Can you work these out from the model? Positions are in its coordinate system, mm. A direction names the side the tool comes from. Give positions to 0.01 mm unless a question says otherwise; leave off trailing zeros. Order: outer loops, then holes, each group sorted by start corner. A loop starts at its lowest first (then second) coordinate and runs counter-clockwise, first axis right, second up.
```python
from build123d import *

# Parameters (mm, degrees)
SKETCH1_R           = 2.5
SKETCH1_R_2         = 1.75
BOSS_EXTRUDE1_DEPTH = 4
SKETCH3_R           = 4.75
SKETCH3_R_2         = 1.75
BOSS_EXTRUDE2_DEPTH = 2.5
FILLET1_R           = 3
FILLET2_R           = 15
SKETCH4_R           = 1.75
CUT_EXTRUDE1_DEPTH  = 2.75


with BuildPart() as part:
    # Sketch1 → Boss-Extrude1 (new body)
    with BuildSketch(Plane(origin=(0, 0, 0), x_dir=(1, 0, 0), z_dir=(0, 1, 0))):
        with BuildLine():
            Line((-33.743770102, 11.787151842), (-29.558909379, 8.857749335))
            ThreePointArc((-29.558909379, 8.857749335), (-30.943257909, 1.876678146), (-29.553838003, -5.103385472))
            Line((-29.553838003, -5.103385472), (-33.733356926, -8.013259417))
            ThreePointArc((-33.733356926, -8.013259417), (-34.979887519, -14.973587102), (-28.019559835, -16.220117695))
            Line((-28.019559835, -16.220117695), (-11.208684115, -4.516012477))
            Line((-11.208684115, -4.516012477), (5.907787468, -4.516012477))
            ThreePointArc((5.907787468, -4.516012477), (10.657787468, 0.233987523), (5.907787468, 4.983987523))
            Line((5.907787468, 4.983987523), (-6.587027339, 4.983987523))
            Line((-6.587027339, 4.983987523), (-28.009146659, 19.979471047))
            ThreePointArc((-28.009146659, 19.979471047), (-34.972617983, 18.750623166), (-33.743770102, 11.787151842))
        make_face()
        with Locations((-30.87645838, 15.883311444)):
            Circle(SKETCH1_R, mode=Mode.SUBTRACT)
        with Locations((-30.87645838, -12.116688556)):
            Circle(SKETCH1_R, mode=Mode.SUBTRACT)
        with Locations((-26.092212532, 0.233987523)):
            Circle(SKETCH1_R_2, mode=Mode.SUBTRACT)
        with Locations((5.907787468, 0.233987523)):
            Circle(SKETCH1_R_2, mode=Mode.SUBTRACT)
    extrude(amount=BOSS_EXTRUDE1_DEPTH)

    # Sketch3 → Boss-Extrude2 (add)
    with BuildSketch(Plane(origin=(0, 4, 0), x_dir=(1, 0, 0), z_dir=(0, 1, 0))):
        with Locations((-26.092212532, 0.233987523)):
            Circle(SKETCH3_R)
        with Locations((-26.092212532, 0.233987523)):
            Circle(SKETCH3_R_2, mode=Mode.SUBTRACT)
        with Locations((5.907787468, 0.233987523)):
            Circle(SKETCH3_R)
        with Locations((5.907787468, 0.233987523)):
            Circle(SKETCH3_R_2, mode=Mode.SUBTRACT)
    extrude(amount=BOSS_EXTRUDE2_DEPTH)

    # Fillet1
    fillet1_edges = [part.edges().sort_by_distance(p)[0] for p in [
        (-29.553838003, 2, 5.103385472),
        (-29.558909379, 2, -8.857749335),
    ]]
    fillet(fillet1_edges, radius=FILLET1_R)

    # Fillet2
    fillet2_edges = [part.edges().sort_by_distance(p)[0] for p in [
        (-11.208684115, 2, 4.516012477),
        (-6.587027339, 2, -4.983987523),
    ]]
    fillet(fillet2_edges, radius=FILLET2_R)

    # Sketch4 → Cut-Extrude1 (cut)
    with BuildSketch(Plane.XZ):
        with BuildLine():
            ThreePointArc((-2.629044497, 2.616012477), (-3.092212532, -0.233987523), (-2.629044497, -3.083987523))
            Line((-2.629044497, -3.083987523), (9.707787468, -3.083987523))
            ThreePointArc((9.707787468, -3.083987523), (10.657787468, -0.233987523), (9.707787468, 2.616012477))
            Line((9.707787468, 2.616012477), (-2.629044497, 2.616012477))
        make_face()
        with Locations((5.907787468, -0.233987523)):
            Circle(SKETCH4_R, mode=Mode.SUBTRACT)
        with BuildLine():
            Line((-30.90374362, -3.083987523), (-17.555380567, -3.083987523))
            ThreePointArc((-17.555380567, -3.083987523), (-17.092212532, -0.233987523), (-17.555380567, 2.616012477))
            Line((-17.555380567, 2.616012477), (-30.380287253, 2.616012477))
            ThreePointArc((-30.380287253, 2.616012477), (-30.866740114, -0.213350056), (-30.90374362, -3.083987523))
        make_face()
        with Locations((-26.092212532, -0.233987523)):
            Circle(SKETCH4_R, mode=Mode.SUBTRACT)
    extrude(amount=-CUT_EXTRUDE1_DEPTH, mode=Mode.SUBTRACT)


solid = part.part
```
1) Which directions (+Z, -Z, +X, -X, +Y, -Y) give clear straight access to the entire face, cutting with the end or side of a thin tool? Please do faces 1 (the face through (-24, 2.75, 0)), 2 (the face through (-21.704, 5.232, 1.585)), 3 (the face through (-32.559, 1.972, 7.195)).
2) Suppose I cut it at C-C (y = 5.5). Please give me the cut outline in (x, z).
3) Suppose I cut it at D-D (y = 1.5). Please give me the cut outline in (x, z).
4) We'd pull the mould along X, two halves only. Please class faces 4 (the face through (-19.9, 0, -3.4)), 5 (the face through (10.1, 3.9, 2)), 6 (the face through (-35.042, 1.972, 14.883)): +X half, -X half, draft (parallel to the pull), parting line (faces both ways), or undercut.
5) Suppose I cut it at B-B (x = -26). Please give me the cut outline in (y, z).
6) If I drill on line 1 (X direction, y = 6, z = 1); line 2 (Y direction, x = -25, z = -14); line 3 (Z direction, x = 3, y = 3.75), over which ranges is the centre line in solid material (lowest first)?
7) Suppose I cut it at A-A (z = -17.5). Please give me the cut outline in (x, y), and give its area (3 significant figures).
8) I'm going to push flat-ended pins straight in: pin 1 Ø8 at (x, z) = (-30.88, 12.12) entering from +Y; pin 2 Ø3 at (x, y) = (-23.5, 1.5) entering from -Z; pin 3 Ø2 at (x, y) = (-16, 3) entering from +Z; pin 4 Ø3 at (x, z) = (-30.88, -15.88) entering from +Y. Where does each tip first touch, or does it pass through?
Results:
1. face 1: -X, -Y
1. face 2: +Y
1. face 3: -X, +Y, -Y
2. outline: circle Ø9.5 at (-26.09, -0.23); circle Ø9.5 at (5.91, -0.23); hole circle Ø3.5 at (-26.09, -0.23); hole circle Ø3.5 at (5.91, -0.23)
3. outline: (-33.74, -11.79) arc R5 ccw to (-28.01, -19.98) - (-10.46, -7.7) arc R15 cw to (-1.86, -4.98) - (5.91, -4.98) arc R4.75 ccw to (9.71, -3.08) - (-2.63, -3.08) arc R9 cw to (-2.63, 2.62) - (9.71, 2.62) arc R4.75 ccw to (5.91, 4.52) - (-6.5, 4.52) arc R15 cw to (-15.07, 7.21) - (-28.02, 16.22) arc R5 ccw to (-33.73, 8.01) - (-31.42, 6.4) arc R3 cw to (-30.25, 3.12) arc R18.26 ccw to (-30.38, 2.62) - (-17.56, 2.62) arc R9 cw to (-17.56, -3.08) - (-30.9, -3.08) arc R18.26 ccw to (-30.25, -6.88) arc R3 cw to (-31.41, -10.16) - close; hole circle Ø5 at (-30.88, -15.88); hole circle Ø5 at (-30.88, 12.12)
4. face 4: draft
4. face 5: undercut
4. face 6: parting line
5. outline: (0, -18.57) - (4, -18.57) - (4, -4.98) - (6.5, -4.98) - (6.5, -1.98) - (2.75, -1.98) - (2.75, -3.08) - (0, -3.08) - close; (0, 2.62) - (2.75, 2.62) - (2.75, 1.51) - (6.5, 1.51) - (6.5, 4.52) - (4, 4.52) - (4, 14.81) - (0, 14.81) - close
6. line 1: x = -30.68 to -27.33, -24.85 to -21.51, 1.32 to 4.67, 7.15 to 10.49
6. line 2: y = 0 to 4
6. line 3: z = -4.98 to 4.52
7. outline: (-35.61, 0) - (-32.78, 0) - (-32.78, 4) - (-35.61, 4) - close; (-28.97, 0) - (-24.47, 0) - (-24.47, 4) - (-28.97, 4) - close
7. area: 29.3 mm2
8. pin 1: stops at y = 4
8. pin 2: stops at z = -17.87
8. pin 3: stops at z = 8.55
8. pin 4: passes through
